CAD build for the part. Positions are in the model's coordinates, mm. Face numbers are marked on the shaded views. A direction names the side the tool comes from. Coordinates: 2 decimals unless noted, no trailing zeros. Order: outer loops, then holes, each group sorted by start corner. A loop starts at its lowest first (then second) coordinate and runs counter-clockwise, first axis right, second up. Notation, with made-up numbers: (19, 44) - (75, 44) arc R34 cw to (75, 83) - close; hole circle Ø2 at (79.25, 69.5). An arc over 180 degrees is marked (long way). Return JSON: item names as keys, results as strings.
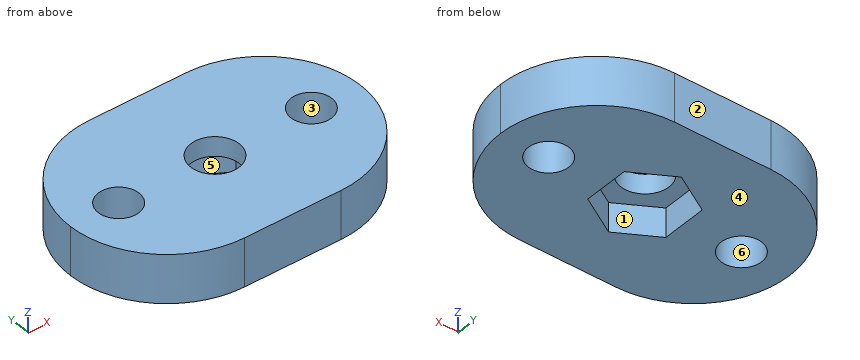
from build123d import *

# Parameters (mm, degrees)
F0_R     = 2.1
F0_R_2   = 2.5
F1_DEPTH = 5
F2_R     = 9.99999
F3_R     = 2.5
F4_DEPTH = 3


# Not quite as in the source:
# - a fillet or chamfer is up to 0.001 mm smaller than in the source, because OpenCascade refuses the exact size


with BuildPart() as f1:
    # F0 (on Top) → F1 (new body)
    with BuildSketch(Plane.XY):
        Polygon((0, 0), (-20, 0), (-25, 0), (-25, -20), (-20, -20), (0, -20), (5, -20), (5, 0), align=None)
        with Locations((-20, -10)):
            Circle(F0_R, mode=Mode.SUBTRACT)
        with Locations((-10, -10)):
            Circle(F0_R_2, mode=Mode.SUBTRACT)
        with Locations((0, -10)):
            Circle(F0_R, mode=Mode.SUBTRACT)
    extrude(amount=F1_DEPTH)

    # F2 (radius 10 in the source; OpenCascade refuses exactly that, so slightly less here)
    f2_edges = [f1.edges().sort_by_distance(p)[0] for p in [
        (-25, -20, 2.5),
        (5, -20, 2.5),
        (5, 0, 2.5),
        (-25, 0, 2.5),
    ]]
    fillet(f2_edges, radius=F2_R)

    # F3 (on face) → F4 (cut)
    with BuildSketch(Plane(origin=(0, 0, 0), x_dir=(1, 0, 0), z_dir=(0, 0, -1))):
        Polygon((-14.05, 12.3382685902), (-14.05, 7.6617314098), (-10, 5.3234628196), (-5.95, 7.6617314098), (-5.95, 12.3382685902), (-10, 14.6765371804), align=None)
        with Locations((-10, 10)):
            Circle(F3_R, mode=Mode.SUBTRACT)
        with Locations((-10, 10)):
            Circle(F3_R)
    extrude(amount=-F4_DEPTH, mode=Mode.SUBTRACT)


solid = f1.part
Item 1: Band-saw the part on A-A, the plane z = 4.25. Count the separate pieces of the cut face and the enclosed holes in it, then the cut area to 3 significant figures.
Findings below:
{"separate pieces": "1", "enclosed holes": "3", "area": "467 mm²"}
Item 2: Band-saw the part on B-B, the plane x = -9.5. List the corners of the cut face in (y, z).
Findings below:
{"outline": "(-20, 0) - (-14.39, 0) - (-14.39, 3) - (-12.45, 3) - (-12.45, 5) - (-20, 5) - close; (-7.55, 3) - (-5.61, 3) - (-5.61, 0) - (0, 0) - (0, 5) - (-7.55, 5) - close"}
Item 3: Mould opens along Y. For the marked faces 1, 2, 3 and 4 say: released by +Y, released by -Y, zero draft, split by the parting line, or undercut.
Findings below:
{"face 1": "undercut", "face 2": "released by +Y", "face 3": "undercut", "face 4": "zero draft"}
Item 4: Wall check: L1, parallel to X at y = -9, z = 3.5; L2, parallel to Z at x = -12.5, y = -8.5; L3, parallel to X at y = -14.5, z = 0.75. Give the ranges that are in metal, low to high. Write a range as [from, to].
Findings below:
{"L1": "x = [-24.95, -21.85], [-18.15, -12.29], [-7.71, -1.85], [1.85, 4.95]", "L2": "z = [3, 5]", "L3": "x = [-23.93, -10.31], [-9.69, 3.93]"}
Item 5: Drop flat-ended pins along their axis: P1, Ø1, axis at y = -6.5, z = 2, coming from the -X side; P2, Ø2.5, axis at x = 0, y = -10, coming from the -Z side; P3, Ø1, axis at y = -6.5, z = 0.5, coming from the +X side. Give the stop position or say it passes through.
Findings below:
{"P1": "stops at x = -24.54", "P2": "passes through", "P3": "stops at x = 4.54"}
Item 6: Band-saw the part on C-C, the plane y = -9.5. List the corners of the cut face in (x, z), then the cut area to 3 significant figures.
Findings below:
{"outline": "(-24.99, 0) - (-22.04, 0) - (-22.04, 5) - (-24.99, 5) - close; (-17.96, 0) - (-14.05, 0) - (-14.05, 3) - (-12.45, 3) - (-12.45, 5) - (-17.96, 5) - close; (-7.55, 3) - (-5.95, 3) - (-5.95, 0) - (-2.04, 0) - (-2.04, 5) - (-7.55, 5) - close; (2.04, 0) - (4.99, 0) - (4.99, 5) - (2.04, 5) - close", "area": "75.0 mm²"}
Item 7: Which spindle directions (+Z, -Z, +X, -X, +Y, -Y) get a long thin tool onto all of the face, cutting with end or side? Do the marked faces 5 and 6. Say none if no direction does.
Findings below:
{"face 5": "-Z", "face 6": "+Z, -Z"}
